```python
from build123d import *

# Parameters (mm, degrees)
CHAMFER_1_SIZE           = 2
CUT_EXTRUDE_1_DEPTH      = 28.184554438
CUT_EXTRUDE_1_DEPTH_BACK = 28.184554438
SKETCH_2_R               = 5.5
CUT_EXTRUDE_2_DEPTH      = 25.372115214
CUT_EXTRUDE_2_DEPTH_BACK = 25.372115214
SKETCH_3_OUTSIDE_W       = 41.142
SKETCH_3_OUTSIDE_H       = 41.142


with BuildPart() as part:
    # 草图1 → 旋转1 (revolve)
    with BuildSketch(Plane(origin=(0, 0, 0), x_dir=(0, 0, -1), z_dir=(1, 0, 0))):
        Polygon((-17, 0), (-17, 12), (-7, 12), (-7, 10), (-5, 10), (-5, 15), (0, 15), (0, 0), align=None)
    revolve(axis=Axis((0, 0, 0), (0, 0, 1)))

    # 倒角1
    chamfer_1_edges = [part.edges().sort_by_distance(p)[0] for p in [
        (0, -15, 0),
    ]]
    chamfer(chamfer_1_edges, length=CHAMFER_1_SIZE)

    # 草图2 → 切除-拉伸1 (cut, two sides: drawn at the far end of the back side and taken through both)
    with BuildSketch(Plane.XY.offset(17).offset(-CUT_EXTRUDE_1_DEPTH_BACK)):
        Circle(SKETCH_2_R)
    extrude(amount=CUT_EXTRUDE_1_DEPTH + CUT_EXTRUDE_1_DEPTH_BACK, mode=Mode.SUBTRACT)

    # 草图3 outside → 切除-拉伸2 (cut, two sides: drawn at the far end of the back side and taken through both)
    with BuildSketch(Plane.XY.offset(5).offset(-CUT_EXTRUDE_2_DEPTH_BACK)):
        Rectangle(SKETCH_3_OUTSIDE_W, SKETCH_3_OUTSIDE_H)
        Polygon((0, 15), (-12.990381057, 7.5), (-12.990381057, -7.5), (0, -15), (12.990381057, -7.5), (12.990381057, 7.5), align=None, mode=Mode.SUBTRACT)
    extrude(amount=CUT_EXTRUDE_2_DEPTH + CUT_EXTRUDE_2_DEPTH_BACK, mode=Mode.SUBTRACT)


solid = part.part
```
Design review of the part built by this model. Coordinates are the model's own, in mm. A direction names the side the tool comes from. Coordinates: 2 decimals unless noted, no trailing zeros. Write each loop counter-clockwise with the first axis right and the second up, starting at its lowest first coordinate (ties: lowest second). Pieces come first, ordered by that corner, then holes.
1) Add section D-D (z = 5.75). Write out the cut boundary in (x, y), plus the area to 3 significant figures.
2) Add section C-C (z = 12.5). Write out the cut boundary in (x, y), plus the area to 3 significant figures.
3) Mouldability with a two-part tool opening along Y and no side actions: class faces 4 (the flat face through (-6.586, -11.198, 3.021)), 5 (the cylindrical face through (-1.19, -5.37, 8.38)), 6 (the flat face through (2.5, -5.2, 17)) as +Y half, -Y half, draft (parallel to the pull), parting line (faces both ways), or undercut.
4) Add section B-B (y = 0). Write out the cut boundary in (x, z).
5) To check wall thickness, follow L1, parallel to Z at x = -1.5, y = 10; L2, parallel to Y at x = 0, z = 10.25. State the ranges of each line that lie inside material, in increasing order.
6) Add section A-A (z = 3). Write out the cut boundary in (x, y).
7) Insertion check: pin 1 (1 mm diameter, centred on x = -10.5, z = 5, fed in from -Y); pin 2 (1.5 mm diameter, centred on x = -3.5, z = 13.5, fed in from +Y); pin 3 (8 mm diameter, centred on y = 8, z = 9.5, fed in from +X). Each pin has a flat end and moves straight along its axis. Give the tip position at first contact, or say it passes through.
8) Machinability: for faces 1 (the cylindrical face through (-0.53, -11.99, 11.93)), 2 (the conical face through (-11.75, -6.75, 0.55)), 3 (the flat face through (-9, -5, 7)), which of the approach directions +Z, -Z, +X, -X, +Y, -Y give a long, thin tool a straight path to every point of the face, cutting with its end or side? Answer none if there is none.
Check result:
1. outline: circle Ø20 at (0, 0); hole circle Ø11 at (0, 0)
1. area: 219 mm2
2. outline: circle Ø24 at (0, 0); hole circle Ø11 at (0, 0)
2. area: 357 mm2
3. face 4: -Y half
3. face 5: undercut
3. face 6: draft
4. outline: (-12.99, 0) - (-5.5, 0) - (-5.5, 17) - (-12, 17) - (-12, 7) - (-10, 7) - (-10, 5) - (-12.99, 5) - close; (5.5, 0) - (12.99, 0) - (12.99, 5) - (10, 5) - (10, 7) - (12, 7) - (12, 17) - (5.5, 17) - close
5. L1: z = 0 to 5, 7 to 17
5. L2: y = -12 to -5.5, 5.5 to 12
6. outline: (-12.99, -7.5) - (0, -15) - (12.99, -7.5) - (12.99, 7.5) - (0, 15) - (-12.99, 7.5) - close; hole circle Ø11 at (0, 0)
7. pin 1: stops at y = -9.23
7. pin 2: stops at y = 11.68
7. pin 3: stops at x = 11.31
8. face 1: +Z
8. face 2: -Z, -X, -Y
8. face 3: none
